Autodesk Inventor part; units mm, degrees
ref_plane "YZ Plane" through (0, 0, 0) normal (1, 0, 0) x (0, 1, 0)
ref_plane "XZ Plane" through (0, 0, 0) normal (0, 1, 0) x (-1, 0, 0)
ref_plane "XY Plane" through (0, 0, 0) normal (0, 0, 1) x (1, 0, 0)
sketch "Sketch1" plane through (0, 0, 0) normal (0, 1, 0) x (-1, 0, 0)
  line L0 (4.6863, 62.0394) -> (4.6863, 67.0394)
  line L1 (4.6863, 67.0394) -> (54.6863, 67.0394)
  line L2 (54.6863, 67.0394) -> (54.6863, 62.0394)
  line L3 (74.6863, 62.0394) -> (54.6863, 62.0394)
  line L4 (-65.3137, 62.0394) -> (-65.3137, 67.0394)
  line L5 (-65.3137, 67.0394) -> (-115.3137, 67.0394)
  line L6 (-115.3137, 67.0394) -> (-115.3137, 62.0394)
  line L7 (4.6863, 62.0394) -> (-65.3137, 62.0394)
  line L8 (-115.3137, 62.0394) -> (-135.3137, 62.0394)
  circle A0 centre (15.4931, 7.0394) radius 35
  line L9 (-135.3137, -47.9606) -> (-115.3137, -47.9606)
  line L10 (-65.3137, -47.9606) -> (4.6863, -47.9606)
  line L11 (54.6863, -47.9606) -> (74.6863, -47.9606)
  line L12 (79.6863, -10.4606) -> (74.6863, -10.4606)
  line L13 (74.6863, -10.4606) -> (74.6863, -47.9606)
  line L14 (79.6863, -10.4606) -> (79.6863, 24.5394)
  line L15 (79.6863, 24.5394) -> (74.6863, 24.5394)
  line L16 (74.6863, 24.5394) -> (74.6863, 62.0394)
  line L17 (-140.3137, -10.4606) -> (-140.3137, 24.5394)
  line L18 (-140.3137, -10.4606) -> (-135.3137, -10.4606)
  line L19 (-135.3137, -10.4606) -> (-135.3137, -47.9606)
  line L20 (-140.3137, 24.5394) -> (-135.3137, 24.5394)
  line L21 (-135.3137, 24.5394) -> (-135.3137, 62.0394)
  line L22 (-115.3137, -47.9606) -> (54.6863, -47.9606)
  circle A1 centre (50.9931, -28.4606) radius 2.5
  circle A2 centre (-20.0069, -28.4606) radius 2.5
  circle A3 centre (-20.0069, 42.5394) radius 2.5
  circle A4 centre (50.9931, 42.5394) radius 2.5
  line L23 (-112.0454, -9.184) -> (-112.0454, -9.084)
  circle A5 centre (-109.5454, -7.8815) radius 1.5
  circle A6 centre (-109.5454, 22.0394) radius 1.5
  circle A7 centre (-34.5454, 22.0394) radius 1.5
  circle A8 centre (-34.5454, -7.8815) radius 1.5
  point P0 (0, 0)
  dimension "d6" = 50
  dimension "d7" = 5
  dimension "d9" = 50
  dimension "d10" = 5
  dimension "d12" = 70
  dimension "d13" = 50
  dimension "d29" = 70
  dimension "d44" = 5
  dimension "d45" = 5
  dimension "d46" = 5
  dimension "d47" = 5
  dimension "d57" = 3
  dimension "d60" = 3
  dimension "d63" = 3
  dimension "d64" = 3
extrude "Extrusion4" add sketch "Sketch1" along normal blind 5
properties part number "Part Sisi 1"
Here's how the part is built. I have some questions about the finished solid (model axes, mm). A direction names the side the tool comes from. Round coordinates to 2 decimals unless told otherwise and drop trailing zeros. Order: outer loops, then holes, each group sorted by start corner. A loop starts at its lowest first (then second) coordinate and runs counter-clockwise, first axis right, second up. Notation, with made-up numbers: M -7,-23 L 27,-23 A21 ccw 27,4 Z; hole C 68.5,36.5 d8. An arc over 180 degrees is marked long. Return JSON: item names as keys, results as strings. Group by question number.
1. If we section it at D-D on x = -59.5: List the corners of the cut face in (y, z) for me, then the cut area to 3 significant figures.
2. If we mould it in two halves opening along Z, with no side actions, what happens to faces 1 (the face through (-29, 2, 67.039)), 2 (the face through (-54.686, 2, 65)), 3 (the face through (20.55, 2.46, 44.98))? For each: pulls with the +Z half, pulls with the -Z half, needs draft (parallel to the pull), parting line crosses it, or undercut.
3. If we section it at B-B on z = -13.5: List the corners of the cut face in (x, y) for me.
4. If we section it at C-C on y = 2.9: State how many separate pieces and enclosed holes the cut face has, then the cut area to 3 significant figures.
5. If we section it at A-A on x = 0: List the corners of the cut face in (y, z) for me.
6. On a 3-axis mill with a long thin cutter (end or side, diameter ignored), from which of +Z, -Z, +X, -X, +Y, -Y can I reach the whole of each face in a straight line? I mean faces 4 (the face through (30, 2, 62.039)), 5 (the face through (138, 2, -10.461)), 6 (the face through (135.314, 2, 43)), 7 (the face through (-65, 2, 62.039)). Say none if no direction works.
7. Please list where these lines run through material, in increasing order: probe 1 along X at (y, z) = (3.25, -8.5); probe 2 along X at (y, z) = (2.65, 43.5); probe 3 along X at (y, z) = (2.7, -41.5).
8. I'm going to push flat-ended pins straight in: pin 1 Ø2.5 at (y, z) = (2.5, 39) entering from -X; pin 2 Ø2.5 at (y, z) = (2, -33) entering from +X; pin 3 Ø2.5 at (x, y) = (39, 2.5) entering from +Z. Where does each tip first touch, or does it pass through?
Reply:
{
 "1": {"outline": "M 0,-47.96 L 5,-47.96 L 5,62.04 L 0,62.04 Z", "area": "550 mm^2"},
 "2": {"face 1": "pulls with the +Z half", "face 2": "needs draft", "face 3": "undercut"},
 "3": {"outline": "M -74.69,0 L -43.83,0 L -43.83,5 L -74.69,5 Z; M 12.85,0 L 135.31,0 L 135.31,5 L 12.85,5 Z"},
 "4": {"separate pieces": "1", "enclosed holes": "9", "area": "20,000 mm^2"},
 "5": {"outline": "M 0,-47.96 L 5,-47.96 L 5,-24.34 L 0,-24.34 Z; M 0,38.42 L 5,38.42 L 5,62.04 L 0,62.04 Z"},
 "6": {"face 4": "+Z, +Y, -Y", "face 5": "-Z, +X, +Y, -Y", "face 6": "+Z, +X, +Y, -Y", "face 7": "+Z, -X, +Y, -Y"},
 "7": {"probe 1": "-79.69 to -46.85, 15.87 to 33.18, 35.91 to 108.18, 110.91 to 140.31", "probe 2": "-74.69 to -53.3, -48.69 to 17.7, 22.31 to 135.31", "probe 3": "-74.69 to 135.31"},
 "8": {"pin 1": "x = -74.69", "pin 2": "x = 135.31", "pin 3": "z = 62.04"}
}
